The drawing under review shows one solid part. Ordinate dimensions are in mm from its lowest x, y, z. A direction names the side the tool comes from. Round coordinates to 2 decimals unless told otherwise and drop trailing zeros. Order: outer loops, then holes, each group sorted by start corner. A loop starts at its lowest first (then second) coordinate and runs counter-clockwise, first axis right, second up. Notation, with made-up numbers: M 71.5,44 L 84.5,44 A9 ccw 84.5,53 Z; hole C 41.25,38.25 d1. An arc over 180 degrees is marked long. Answer as a JSON object with one key per item and string values. Group by question number.
1. To check wall thickness, follow probe 1 along Y at (x, z) = (7, 10.85); probe 2 along Y at (x, z) = (45, 10.45); probe 3 along Z at (x, y) = (4.5, 28.5). State the ranges of each line that lie inside material, in increasing order. Write a range as [from, to].
2. Add section A-A on x = 7. State the section outline as (y, z) points, and give its area (3 significant figures).
3. Machinability: for the marked faces 1, 2 and 3, which of the approach directions +Z, -Z, +X, -X, +Y, -Y give a long, thin tool a straight path to every point of the face, cutting with its end or side? Answer none if there is none.
4. Add section D-D on x = 25. State the section outline as (y, z) points.
5. Clearance check with flat-ended pins moving along their axes: P1, Ø10, axis at x = 6, z = 23, coming from the -Y side; P2, Ø4, axis at x = 34.5, y = 33, coming from the +Z side; P3, Ø8, axis at y = 35, z = 4.5, coming from the -X side. State where each tip first meets the part, or that it passes through.
6. Add section C-C on y = 35. State the section outline as (x, z) points.
7. Add section B-B on y = 7. State the section outline as (x, z) points, and give its area (3 significant figures).
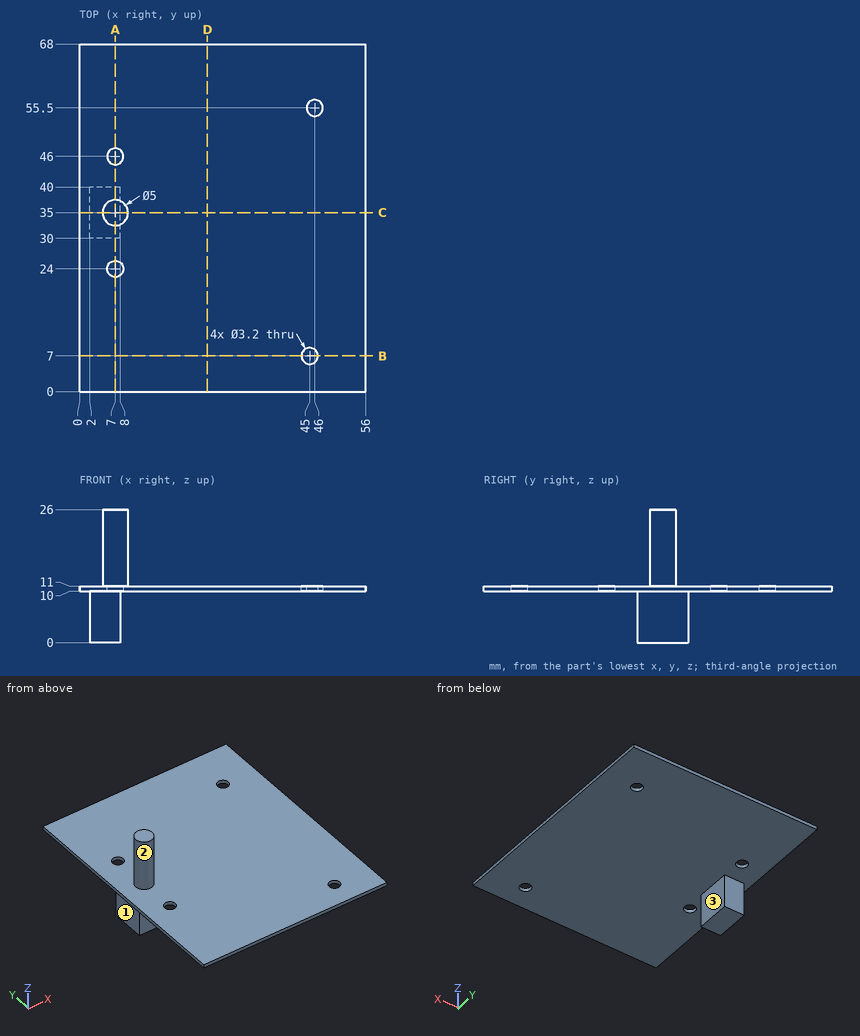
Recorded:
{
 "1": {"probe 1": "y = [0, 22.4], [25.6, 44.4], [47.6, 68]", "probe 2": "y = [0, 5.4], [8.6, 54.25], [56.75, 68]", "probe 3": "z = [10, 11]"},
 "2": {"outline": "M 0,10 L 22.4,10 L 22.4,11 L 0,11 Z; M 25.6,10 L 30,10 L 30,0 L 40,0 L 40,10 L 44.4,10 L 44.4,11 L 37.5,11 L 37.5,26 L 32.5,26 L 32.5,11 L 25.6,11 Z; M 47.6,10 L 68,10 L 68,11 L 47.6,11 Z", "area": "237 mm²"},
 "3": {"face 1": "-Z, -X, +Y, -Y", "face 2": "+Z", "face 3": "-Z, +X, +Y, -Y"},
 "4": {"outline": "M 0,10 L 68,10 L 68,11 L 0,11 Z"},
 "5": {"P1": "stops at y = 32.5", "P2": "stops at z = 11", "P3": "stops at x = 2"},
 "6": {"outline": "M 0,10 L 2,10 L 2,0 L 8,0 L 8,10 L 56,10 L 56,11 L 9.5,11 L 9.5,26 L 4.5,26 L 4.5,11 L 0,11 Z"},
 "7": {"outline": "M 0,10 L 43.4,10 L 43.4,11 L 0,11 Z; M 46.6,10 L 56,10 L 56,11 L 46.6,11 Z", "area": "52.8 mm²"}
}
